Design review of the part shown in the three views and the two pictorial views. Dimensions are in mm from the part's minimum x, y and z. A direction names the side the tool comes from. Round coordinates to 2 decimals unless told otherwise and drop trailing zeros. Order: outer loops, then holes, each group sorted by start corner. A loop starts at its lowest first (then second) coordinate and runs counter-clockwise, first axis right, second up.
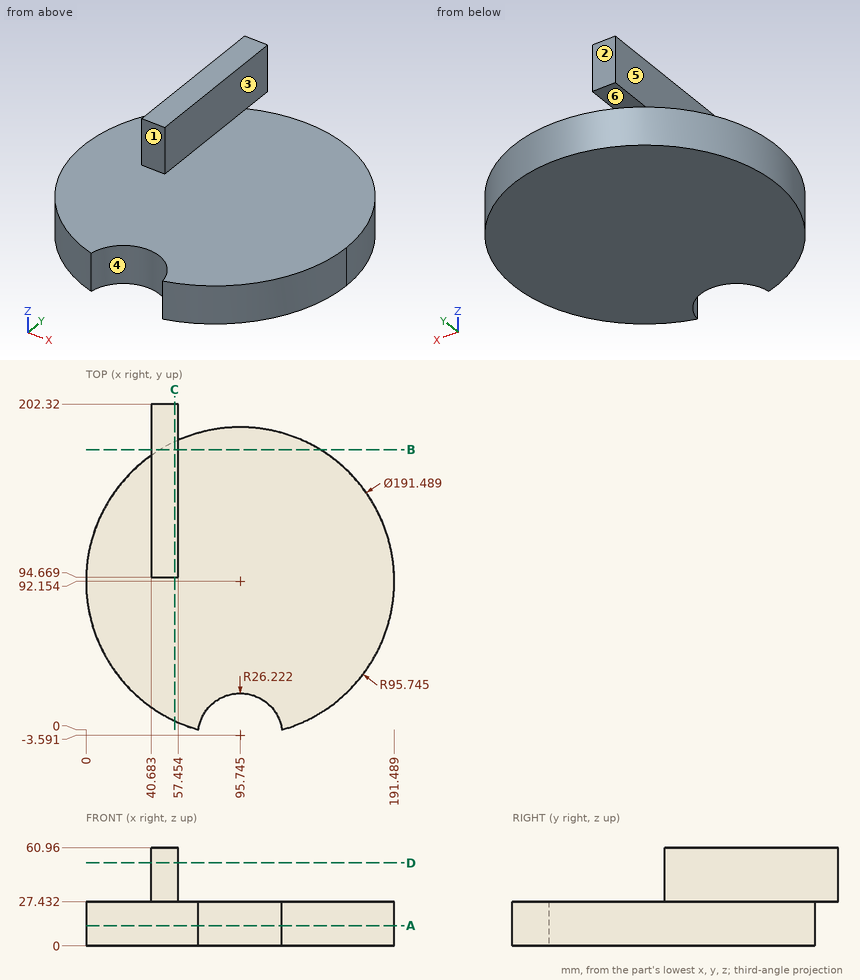
(1) Consider section B-B (y = 174). Write out the cut boundary in (x, z) (1 decimal), and give its area (3 significant figures).
Data:
outline: (40.7, 27.4) - (46.1, 27.4) - (46.1, 0) - (145.4, 0) - (145.4, 27.4) - (57.5, 27.4) - (57.5, 61) - (40.7, 61) - close
area: 3,290 mm2
(2) To check wall thickness, follow probe 1 along Z at (x, y) = (156, 61); probe 2 along X at (y, z) = (126.5, 30); probe 3 along Y at (x, z) = (72, 21) (1 decimal). State the ranges of each line that lie inside material, in increasing order.
Data:
probe 1: z = 0 to 27.43
probe 2: x = 40.68 to 57.45
probe 3: y = 7.5 to 184.9
(3) Consider section C-C (x = 55). Write out the cut boundary in (y, z).
Data:
outline: (5.51, 0) - (178.8, 0) - (178.8, 27.43) - (202.32, 27.43) - (202.32, 60.96) - (94.67, 60.96) - (94.67, 27.43) - (5.51, 27.43) - close
(4) Consider section D-D (z = 51.5). Write out the cut boundary in (x, y).
Data:
outline: (40.68, 94.67) - (57.45, 94.67) - (57.45, 202.32) - (40.68, 202.32) - close
(5) For the marked faces 1 and 2, list the 3-axis set-ups (+Z, -Z, +X, -X, +Y, -Y) from which the entire face can be reached by the end or side of a thin tool; tool diameter is ignored.
Data:
face 1: +Z, +X, -X, -Y
face 2: +Z, -Z, +X, -X, +Y
(6) Consider section A-A (z = 12.5). Write out the cut boundary in (x, y) (1 decimal), and give its area (3 significant figures).
Data:
outline: (69.8, 0) arc R26.2 cw to (121.7, 0) arc R95.7 ccw (long way) to start
area: 27,800 mm2
(7) Insertion check: pin 1 (12 mm diameter, centred on x = 21.5, y = 27.5, fed in from -Z); pin 2 (5 mm diameter, centred on x = 153.5, z = 12, fed in from +Y) (1 decimal); pin 3 (10 mm diameter, centred on x = 53.5, z = 8.5, fed in from -Y); pin 4 (1 mm diameter, centred on x = 161, z = 27, fed in from -Y). Each pin has a flat end and moves straight along its axis. Give the tip position at first contact, or say it passes through.
Data:
pin 1: stops at z = 0
pin 2: stops at y = 170.3
pin 3: stops at y = 3.95
pin 4: stops at y = 21.63
(8) Draft analysis for pull direction X (two halves, no side actions). For the marked faces 3, 4, 5 and 6, state which applies: pulls with the +X half, pulls with the -X half, needs draft (parallel to the pull), parting line crosses it, or undercut.
Data:
face 3: pulls with the +X half
face 4: undercut
face 5: pulls with the -X half
face 6: needs draft
